Could you check a few things on this model? Use its own coordinates, in mm. A direction names the side the tool comes from. Round coordinates to 2 decimals unless told otherwise and drop trailing zeros. Loops run counter-clockwise (first coordinate to the right, second up) from the corner with the lowest first, then second, coordinate; pieces in that order, holes last. Notation, with made-up numbers: M -34.75,41 L -10.75,41 A6 ccw -10.75,52 Z; hole C -21.5,12 d9. An arc over 180 degrees is marked long. Answer in a Markdown table with one row per item.
Autodesk Inventor part; units mm, degrees
ref_plane "Work Plane2" through (0, 6.35, 0) normal (0, 1, 0) x (1, 0, 0)
ref_plane "YZ Plane" through (0, 0, 0) normal (1, 0, 0) x (0, 1, 0)
ref_plane "XZ Plane" through (0, 0, 0) normal (0, 1, 0) x (-1, 0, 0)
sketch "Sketch1" plane through (0, 0, 0) normal (0, 0, 1) x (1, 0, 0)
  circle A0 centre (0, 0) radius 5.715
  circle A1 centre (0, 0) radius 5.08
  line L0 (0, 0) -> (5.715, 0)
  dimension "d0" = 11.43
  dimension "d1" = 10.16
extrude "Extrusion1" add sketch "Sketch1" along normal blind 50.8
sketch "Sketch2" plane through (0, 0, 50.8) normal (0, 0, 1) x (1, 0, 0)
  circle A0 centre (0, 0) radius 5.08
  circle A1 centre (0, 0) radius 5.715
  circle A2 centre (0, 0) radius 7.62
  dimension "d4" = 15.24
extrude "Extrusion2" add sketch "Sketch2" along normal blind 1.27 contours A1 | A2
ref_plane "Work Plane2" through (0, 6.35, 0) normal (0, 1, 0) x (1, 0, 0)
ref_plane "Work Plane1" through (0, 0, 0) normal (0, 1, 0) x (1, 0, 0)
sketch "Sketch3" plane through (0, 6.35, 0) normal (0, 1, 0) x (1, 0, 0)
  line L0 (0, 0) -> (0, -5.08)
  circle A0 centre (0, -5.08) radius 2.54
  dimension "d9" = 5.08
  dimension "d10" = 5.08
extrude "Extrusion3" cut sketch "Sketch3" against normal blind 25.4
properties part number "Pin" material "Steel"
1) Will these pins go through, and if not, where does the flat tip stop? P1, Ø6, axis at x = 4.5, z = 6, coming from the +Y side; P2, Ø8, axis at y = 5.5, z = 36, coming from the +X side; P3, Ø8, axis at y = 0.5, z = 19, coming from the +X side (3 decimals).
Computed:
| item | result |
|---|---|
| P1 | stops at y = 5.47 |
| P2 | stops at x = 5.51 |
| P3 | stops at x = 5.715 |
2) I want a section at A-A, the plane x = 0. Please give me the cut outline in (y, z) (3 decimals).
Computed:
| item | result |
|---|---|
| outline | M -7.62,50.8 L -5.715,50.8 L -5.715,7.62 L -5.08,7.62 L -5.08,52.07 L -7.62,52.07 Z; M -5.715,0 L -5.08,0 L -5.08,2.54 L -5.715,2.54 Z; M 5.08,0 L 5.715,0 L 5.715,2.54 L 5.08,2.54 Z; M 5.08,7.62 L 5.715,7.62 L 5.715,50.8 L 7.62,50.8 L 7.62,52.07 L 5.08,52.07 Z |
3) If we mould it in two halves opening along X, with no side actions, what happens to faces 3 (the face through (2, -5, 52.07)), 4 (the face through (-1.87, -5.05, 3.36)), 5 (the face through (-1.65, 7.44, 51.43))? For each: released by +X, released by -X, zero draft, split by the parting line, or undercut.
Computed:
| item | result |
|---|---|
| face 3 | zero draft |
| face 4 | undercut |
| face 5 | split by the parting line |
4) I want a section at C-C, the plane z = 5.08. Please give me the cut outline in (x, y) (3 decimals), plus the area to 3 significant figures.
Computed:
| item | result |
|---|---|
| outline | M -2.54,-5.12 L -2.54,-4.399 A5.08 cw -2.54,4.399 L -2.54,5.12 A5.715 ccw Z; M 2.54,-5.12 A5.715 ccw 2.54,5.12 L 2.54,4.399 A5.08 cw 2.54,-4.399 Z |
| area | 14.8 mm² |
5) I need wall thicknesses on line 1 (Y direction, x = 0, z = 31.5) (3 decimals); line 2 (Z direction, x = 3.5, y = -6); line 3 (Y direction, x = 3.75, z = 12). Which ranges of each line are inside material? Lowest first, please.
Computed:
| item | result |
|---|---|
| line 1 | y = -5.715 to -5.08, 5.08 to 5.715 |
| line 2 | z = 50.8 to 52.07 |
| line 3 | y = -4.31 to -3.43, 3.43 to 4.31 |
6) I want a section at B-B, the plane y = 0. Please give me the cut outline in (x, z) (3 decimals), plus the area to 3 significant figures.
Computed:
| item | result |
|---|---|
| outline | M -7.62,50.8 L -5.715,50.8 L -5.715,0 L -5.08,0 L -5.08,52.07 L -7.62,52.07 Z; M 5.08,0 L 5.715,0 L 5.715,50.8 L 7.62,50.8 L 7.62,52.07 L 5.08,52.07 Z |
| area | 71.0 mm² |
7) Which directions (+Z, -Z, +X, -X, +Y, -Y) give clear straight access to the entire face, cutting with the end or side of a thin tool? Please do faces 1 (the face through (5.45, -1.72, 25.04)), 2 (the face through (-5, -2, 0)).
Computed:
| item | result |
|---|---|
| face 1 | -Z |
| face 2 | -Z, +X, -X, +Y, -Y |
8) I want a section at D-D, the plane x = 4.5. Please give me the cut outline in (y, z).
Computed:
| item | result |
|---|---|
| outline | M -6.15,50.8 L -3.52,50.8 L -3.52,0 L -2.36,0 L -2.36,52.07 L -6.15,52.07 Z; M 2.36,0 L 3.52,0 L 3.52,50.8 L 6.15,50.8 L 6.15,52.07 L 2.36,52.07 Z |
